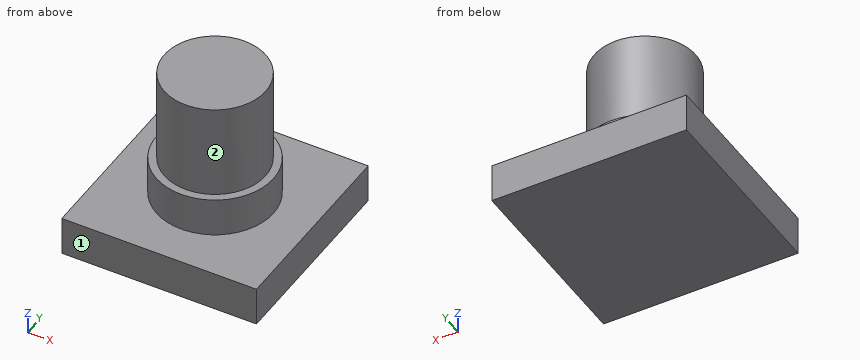
```python
from build123d import *

# Parameters (mm, degrees)
F0_W     = 15
F0_H     = 15
F0_R     = 4.5
F1_DEPTH = 3
F0_R_2   = 3.9
F2_DEPTH = 6
F3_DEPTH = 13.3


with BuildPart() as f1:
    # F0 (on Top) → F1 (new body)
    with BuildSketch(Plane.XY):
        Rectangle(F0_W, F0_H)
        Circle(F0_R, mode=Mode.SUBTRACT)
    extrude(amount=F1_DEPTH)

    # F0 (on Top) → F2 (join)
    with BuildSketch(Plane.XY):
        Circle(F0_R)
        Circle(F0_R_2, mode=Mode.SUBTRACT)
    extrude(amount=F2_DEPTH)

    # F0 (on Top) → F3 (join)
    with BuildSketch(Plane.XY):
        Circle(F0_R_2)
    extrude(amount=F3_DEPTH)


solid = f1.part
```
For this review, take the finished solid that the model builds, in its own axes (mm). Face numbers are marked on the shaded views. A direction names the side the tool comes from. Coordinates: 2 decimals unless noted, no trailing zeros. Order: outer loops, then holes, each group sorted by start corner. A loop starts at its lowest first (then second) coordinate and runs counter-clockwise, first axis right, second up. Notation, with made-up numbers: (2, -29.5) - (14, -29.5) arc R9 cw to (14, -23.5) - close; hole circle Ø2 at (89.25, -25.5). An arc over 180 degrees is marked (long way). Answer as a JSON object with one key per item and string values. Group by question number.
1. Clearance check with flat-ended pins moving along their axes: P1, Ø2, axis at y = 6, z = 6.5, coming from the +X side; P2, Ø4, axis at y = -5, z = 10, coming from the +X side; P3, Ø1.5, axis at x = -1.5, z = 11, coming from the +Y side. State where each tip first meets the part, or that it passes through.
2. For probe 1 along Z at (x, y) = (-5.25, -5); probe 2 along Y at (x, z) = (2.5, 11.5); probe 3 along X at (y, z) = (-1.25, 12.5), list the stretches that pass through material, from the lowest coordinate up.
3. For the marked faces 1 and 2, list the 3-axis set-ups (+Z, -Z, +X, -X, +Y, -Y) from which the entire face can be reached by the end or side of a thin tool; tool diameter is ignored.
4. We need section A-A on y = 0. State the section outline as (x, z) points, then the cut area to 3 significant figures.
5. We need section D-D on y = -4.75. State the section outline as (x, z) points.
6. We need section C-C on z = 11.75. State the section outline as (x, y) points, then the cut area to 3 significant figures.
Final values:
{
 "1": {"P1": "through", "P2": "x = 2.49", "P3": "y = 3.83"},
 "2": {"probe 1": "0 to 3", "probe 2": "-2.99 to 2.99", "probe 3": "-3.69 to 3.69"},
 "3": {"face 1": "+Z, -Z, +X, -X, -Y", "face 2": "+Z"},
 "4": {"outline": "(-7.5, 0) - (7.5, 0) - (7.5, 3) - (4.5, 3) - (4.5, 6) - (3.9, 6) - (3.9, 13.3) - (-3.9, 13.3) - (-3.9, 6) - (-4.5, 6) - (-4.5, 3) - (-7.5, 3) - close", "area": "129 mm²"},
 "5": {"outline": "(-7.5, 0) - (7.5, 0) - (7.5, 3) - (-7.5, 3) - close"},
 "6": {"outline": "circle Ø7.8 at (0, 0)", "area": "47.8 mm²"}
}
